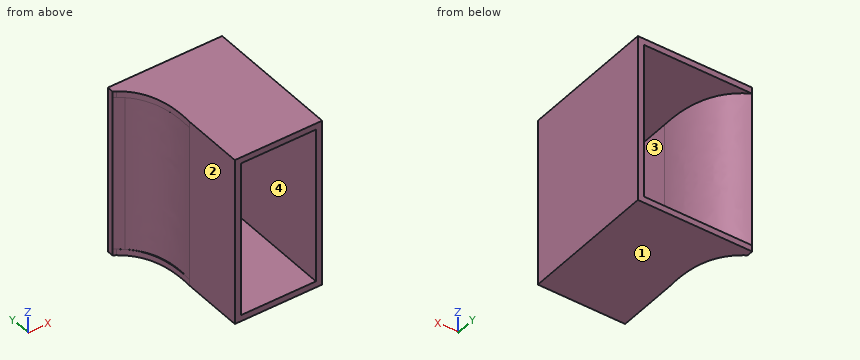
from build123d import *

# Parameters (mm, degrees)
SKETCH7_W               = 25.4
SKETCH7_H               = 303.92823255
BOSS_EXTRUDE2_DEPTH     = 635
BOSS_EXTRUDE2_2_DEPTH   = 635
SKETCH9_W               = 465.483389799
SKETCH9_H               = 303.92823255
BOSS_EXTRUDE3_DEPTH     = 25.4
SKETCH10_W              = 465.483389799
SKETCH10_H              = 303.92823255
BOSS_EXTRUDE4_DEPTH     = 25.4
CUT_EXTRUDE1_DEPTH      = 2380.234
CUT_EXTRUDE1_DEPTH_BACK = 125.476
SKETCH12_W              = 355.6
SKETCH12_H              = 685.8
BOSS_EXTRUDE5_DEPTH     = 254
SKETCH13_W              = 304.8
SKETCH13_H              = 635
CUT_EXTRUDE2_DEPTH      = 551.942


with BuildPart() as part:
    # Sketch7 → Boss-Extrude2 (new body)
    with BuildSketch(Plane.XY):
        with Locations((419.881001745, 151.964116275)):
            Rectangle(SKETCH7_W, SKETCH7_H)
    extrude(amount=BOSS_EXTRUDE2_DEPTH)



with BuildPart() as body_2:
    # Sketch7 → Boss-Extrude2 2 (new body)
    with BuildSketch(Plane.XY):
        with BuildLine():
            Line((-32.902388054, 303.92823255), (-32.902388054, 278.52823255))
            add(Edge.make_bspline(
                [(0, 254), (-15.04510801, 267.251537687), (-32.902388054, 278.52823255)],
                knots=[0.866081735, 0.866081735, 0.866081735, 1, 1, 1], degree=2))
            add(Edge.make_bspline(
                [(76.981001745, 0), (97.30034402, 168.299108064), (0, 254)],
                knots=[0, 0, 0, 0.866081735, 0.866081735, 0.866081735], degree=2))
            Line((76.981001745, 0), (102.381001745, 0))
            add(Edge.make_bspline(
                [(102.381001745, 0), (111.38603621, 225.968646172), (-32.902388054, 303.92823255)],
                knots=[0, 0, 0, 0.936348865, 0.936348865, 0.936348865], degree=2))
        make_face()
    extrude(amount=BOSS_EXTRUDE2_2_DEPTH)


with BuildPart() as part_1:
    add(part.part)

    add(body_2.part)  # Boss-Extrude3 merges body 2
    # Sketch9 → Boss-Extrude3 (add)
    with BuildSketch(Plane.XY.offset(635)):
        with Locations((199.839306846, 151.964116275)):
            Rectangle(SKETCH9_W, SKETCH9_H)
    extrude(amount=BOSS_EXTRUDE3_DEPTH)

    # Sketch10 → Boss-Extrude4 (add)
    with BuildSketch(Plane(origin=(0, 0, 0), x_dir=(-1, 0, 0), z_dir=(0, 0, -1))):
        with Locations((-199.839306846, 151.964116275)):
            Rectangle(SKETCH10_W, SKETCH10_H)
    extrude(amount=BOSS_EXTRUDE4_DEPTH)

    # Sketch11 → Cut-Extrude1 (cut, two sides: drawn at the far end of the back side and taken through both)
    with BuildSketch(Plane(origin=(0, 0, 635), x_dir=(-1, 0, 0), z_dir=(0, 0, -1)).offset(-CUT_EXTRUDE1_DEPTH_BACK)):
        with BuildLine():
            Line((32.902388054, 0), (32.902388054, 278.52823255))
            add(Edge.make_bspline(
                [(32.902388054, 278.52823255), (26.814117535, 274.683550229), (21.052735145, 270.6093113)],
                knots=[0, 0, 0, 0.045658164, 0.045658164, 0.045658164], degree=2))
            add(Edge.make_bspline(
                [(-76.981001745, 0), (-90.995301199, 190.717013874), (21.052735145, 270.6093113)],
                knots=[0, 0, 0, 0.870425908, 0.870425908, 0.870425908], degree=2))
            Line((-76.981001745, 0), (32.902388054, 0))
        make_face()
    extrude(amount=CUT_EXTRUDE1_DEPTH + CUT_EXTRUDE1_DEPTH_BACK, mode=Mode.SUBTRACT)

    # Sketch12 → Boss-Extrude5 (add)
    with BuildSketch(Plane.XZ):
        with Locations((254.781001745, 317.5)):
            Rectangle(SKETCH12_W, SKETCH12_H)
    extrude(amount=BOSS_EXTRUDE5_DEPTH)

    # Sketch13 → Cut-Extrude2 (cut)
    with BuildSketch(Plane(origin=(0, 0, 0), x_dir=(1, 0, 0), z_dir=(0, 1, 0))):
        with Locations((254.781001745, -317.5)):
            Rectangle(SKETCH13_W, SKETCH13_H)
    extrude(amount=-CUT_EXTRUDE2_DEPTH, mode=Mode.SUBTRACT)


solid = part_1.part
The listing builds one solid part. Answer for the finished solid, in the listing's coordinates (mm). Face numbers are marked on the shaded views. Round coordinates to 2 decimals unless told otherwise and drop trailing zeros. Write each loop counter-clockwise with the first axis right and the second up, starting at its lowest first coordinate (ties: lowest second). Pieces come first, ordered by that corner, then holes. Notation, with made-up numbers: (46, 5.5) - (90, 5.5) arc R18 cw to (90, 39.5) - close; hole circle Ø11 at (32, 26). An arc over 180 degrees is marked (long way). Use a Markdown table: item, result. Add a question column.
1. The part is cut by section A-A (x = 303). Write down the section's boundary in (y, z).
2. Flat-ended cylindrical pins translate along their axes: P1, Ø3, axis at y = -149.5, z = 86, coming from the -X side; P2, Ø4, axis at x = 21.5, z = 214.5, coming from the -Y side. Find the tip coordinate at first contact, or state that the pin passes through.
3. Consider line 1 (Z direction, x = 362.5, y = -64); line 2 (X direction, y = -87.5, z = 467); line 3 (X direction, y = 3, z = 143). Determine where each line is inside the solid, lowest interval first.
4. For a pull along X with two mould halves and no side action, classify the marked faces 1, 2, 3 and 4 as +X half, -X half, draft (parallel to the pull), parting line (faces both ways), or undercut.
5. The part is cut by section B-B (y = -158). Write down the section's boundary in (x, z), and give its area (3 significant figures).
Reported:
| question | item | result |
|---|---|---|
| 1 | outline | (-254, -25.4) - (303.93, -25.4) - (303.93, 0) - (-254, 0) - close; (-254, 635) - (303.93, 635) - (303.93, 660.4) - (-254, 660.4) - close |
| 2 | P1 | x = 76.98 |
| 2 | P2 | y = 230.1 |
| 3 | line 1 | -25.4 to 0, 635 to 660.4 |
| 3 | line 2 | 76.98 to 102.38, 407.18 to 432.58 |
| 3 | line 3 | 77.33 to 102.49, 407.18 to 432.58 |
| 4 | face 1 | draft |
| 4 | face 2 | -X half |
| 4 | face 3 | undercut |
| 4 | face 4 | undercut |
| 5 | outline | (76.98, -25.4) - (432.58, -25.4) - (432.58, 660.4) - (76.98, 660.4) - close; hole (102.38, 0) - (407.18, 0) - (407.18, 635) - (102.38, 635) - close |
| 5 | area | 50,300 mm^2 |
